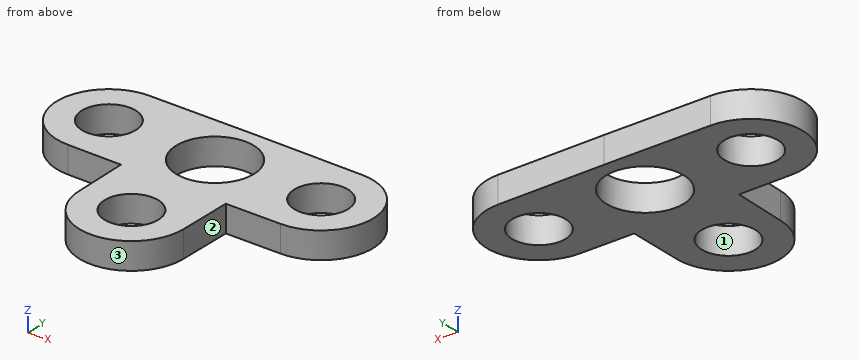
```python
from build123d import *

# Parameters (mm, degrees)
SKETCH3_R           = 3.2
SKETCH3_R_2         = 4.625
BOSS_EXTRUDE1_DEPTH = 3.175


with BuildPart() as part:
    # Sketch3 → Boss-Extrude1 (new body)
    with BuildSketch(Plane.XY):
        with BuildLine():
            Line((0, 6.265082263), (-12.7, 6.2))
            ThreePointArc((-12.7, 6.2), (-18.9, 0), (-12.7, -6.2))
            Line((-12.7, -6.2), (-6.35, -6.232541132))
            Line((-6.35, -6.232541132), (-6.2, -12.7))
            ThreePointArc((-6.2, -12.7), (0, -18.9), (6.2, -12.7))
            Line((6.2, -12.7), (6.2, -6.23330982))
            Line((6.2, -6.23330982), (12.7, -6.2))
            ThreePointArc((12.7, -6.2), (18.9, 0), (12.7, 6.2))
            Line((12.7, 6.2), (0, 6.265082263))
        make_face()
        with Locations((-12.7, 0)):
            Circle(SKETCH3_R, mode=Mode.SUBTRACT)
        with Locations((12.7, 0)):
            Circle(SKETCH3_R, mode=Mode.SUBTRACT)
        Circle(SKETCH3_R_2, mode=Mode.SUBTRACT)
        with Locations((0, -12.7)):
            Circle(SKETCH3_R, mode=Mode.SUBTRACT)
    extrude(amount=BOSS_EXTRUDE1_DEPTH)


solid = part.part
```
The listing builds one solid part. Answer for the finished solid, in the listing's coordinates (mm). Face numbers are marked on the shaded views. Give positions to 0.01 mm unless a question says otherwise; leave off trailing zeros. Write each loop counter-clockwise with the first axis right and the second up, starting at its lowest first coordinate (ties: lowest second). Pieces come first, ordered by that corner, then holes. Notation, with made-up numbers: (-24, -33) -> (23, -33) arc R30 ccw to (23, 0) -> close; hole circle Ø3 at (-24, 3). An arc over 180 degrees is marked (long way). Use one line per item in the form item = value.
1) Section D-D on x = 11 is taken. Write down the section's boundary in (y, z) (3 decimals), plus the area to 3 significant figures.
Result:
outline = (-6.209, 0) -> (-2.711, 0) -> (-2.711, 3.175) -> (-6.209, 3.175) -> close; (2.711, 0) -> (6.209, 0) -> (6.209, 3.175) -> (2.711, 3.175) -> close
area = 22.2 mm²
2) Section A-A on y = 0 is taken. Write down the section's boundary in (x, z) (3 decimals), plus the area to 3 significant figures.
Result:
outline = (-18.9, 0) -> (-15.9, 0) -> (-15.9, 3.175) -> (-18.9, 3.175) -> close; (-9.5, 0) -> (-4.625, 0) -> (-4.625, 3.175) -> (-9.5, 3.175) -> close; (4.625, 0) -> (9.5, 0) -> (9.5, 3.175) -> (4.625, 3.175) -> close; (15.9, 0) -> (18.9, 0) -> (18.9, 3.175) -> (15.9, 3.175) -> close
area = 50.0 mm²
3) Section C-C on x = -12 is taken. Write down the section's boundary in (y, z) (1 decimal), plus the area to 3 significant figures.
Result:
outline = (-6.2, 0) -> (-3.1, 0) -> (-3.1, 3.2) -> (-6.2, 3.2) -> close; (3.1, 0) -> (6.2, 0) -> (6.2, 3.2) -> (3.1, 3.2) -> close
area = 19.6 mm²
4) Section B-B on z = 1.45 is taken. Write down the section's boundary in (x, y) (3 decimals), plus the area to 3 significant figures.
Result:
outline = (-12.7, -6.2) -> (-6.35, -6.233) -> (-6.2, -12.7) arc R6.2 ccw to (6.2, -12.7) -> (6.2, -6.233) -> (12.7, -6.2) arc R6.2 ccw to (12.7, 6.2) -> (0, 6.265) -> (-12.7, 6.2) arc R6.2 ccw to start; hole circle Ø6.4 at (-12.7, 0); hole circle Ø9.25 at (0, 0); hole circle Ø6.4 at (0, -12.7); hole circle Ø6.4 at (12.7, 0)
area = 415 mm²
5) Each of these flat-tipped pins is pushed along its axis until it touches: P1, Ø12, axis at x = 0, y = 0, coming from the +Z side (3 decimals); P2, Ø5, axis at x = 0, y = -12.7, coming from the -Z side; P3, Ø1, axis at y = -9.5, z = 2, coming from the +X side; P4, Ø1, axis at y = -3.5, z = 2, coming from the -X side. Where does it stop, or does it pass through?
Result:
P1 = 3.175
P2 = through
P3 = 6.2
P4 = -18.13
6) Straight lines are drawn through the part: probe 1 along Y at (x, z) = (0, 1.4) (3 decimals); probe 2 along Y at (x, z) = (12.7, 1.75); probe 3 along Y at (x, z) = (1.5, 0.45) (3 decimals). For each, find the intervals that lie inside material, in ascending order.
Result:
probe_1 = -18.9 to -15.9, -9.5 to -4.625, 4.625 to 6.265
probe_2 = -6.2 to -3.2, 3.2 to 6.2
probe_3 = -18.716 to -15.527, -9.873 to -4.375, 4.375 to 6.257
7) For a pull along Y with two mould halves and no side action, classify the marked faces 1, 2 and 3 as +Y half, -Y half, draft (parallel to the pull), parting line (faces both ways), or undercut.
Result:
face_1 = undercut
face_2 = draft
face_3 = -Y half
